```python
from build123d import *

# Parameters (mm, degrees)
BOSS_EXTRUDE1_DEPTH     = 19.05
CUT_EXTRUDE4_DEPTH      = 0.508
CUT_EXTRUDE4_DEPTH_BACK = 6.858
SKETCH4_W               = 31.54
SKETCH4_H               = 60.54
SKETCH4_W_2             = 1.905
SKETCH4_H_2             = 7.62
SKETCH4_3_W             = 1.905
SKETCH4_3_H             = 7.62
CUT_EXTRUDE5_DEPTH      = 34.798
SKETCH5_W               = 31.679207877
SKETCH5_H               = 2.54
SKETCH5_W_2             = 31.841170495
BOSS_EXTRUDE2_DEPTH     = 54.61
SKETCH6_W               = 1.77119272
SKETCH6_H               = 7.149457174
CUT_EXTRUDE6_DEPTH      = 90.782
SKETCH4_5_R             = 1.524
CUT_EXTRUDE7_DEPTH      = 90.782


with BuildPart() as part:
    # Sketch2 → Boss-Extrude1 (new, symmetric)
    with BuildSketch(Plane.XY):
        with BuildLine():
            Line((8.128, -45.72), (8.128, 45.72))
            ThreePointArc((8.128, 45.72), (5.747363917, 51.467363917), (0, 53.848))
            Line((0, 53.848), (0, -53.848))
            ThreePointArc((0, -53.848), (5.747363917, -51.467363917), (8.128, -45.72))
        make_face()
    extrude(amount=BOSS_EXTRUDE1_DEPTH, both=True)

    # Sketch4 → Cut-Extrude4 (cut, two sides: drawn at the far end of the back side and taken through both)
    # profile 1 of 3: a face of its own
    with BuildSketch(Plane.ZY.offset(-CUT_EXTRUDE4_DEPTH_BACK)):
        with Locations((0.025266364, 0.022760685)):
            Rectangle(SKETCH4_W, SKETCH4_H)
        with Locations((-6.375, 9.13)):
            Rectangle(SKETCH4_W_2, SKETCH4_H_2, mode=Mode.SUBTRACT)
        with Locations((6.375, 9.13)):
            Rectangle(SKETCH4_W_2, SKETCH4_H_2, mode=Mode.SUBTRACT)
    # profile 2 of 3: a face of its own
    with BuildSketch(Plane.ZY.offset(-CUT_EXTRUDE4_DEPTH_BACK)):
        with Locations((-6.375, 9.13)):
            Rectangle(SKETCH4_W_2, SKETCH4_H_2)
    # profile 3 of 3: a face of its own
    with BuildSketch(Plane.ZY.offset(-CUT_EXTRUDE4_DEPTH_BACK)):
        with Locations((6.375, 9.13)):
            Rectangle(SKETCH4_W_2, SKETCH4_H_2)
    extrude(amount=CUT_EXTRUDE4_DEPTH + CUT_EXTRUDE4_DEPTH_BACK, mode=Mode.SUBTRACT)

    # Sketch4_3 → Cut-Extrude5 (cut)
    with BuildSketch(Plane.ZY):
        with Locations((-6.375, 9.13)):
            Rectangle(SKETCH4_3_W, SKETCH4_3_H)
        with Locations((6.375, 9.13)):
            Rectangle(SKETCH4_3_W, SKETCH4_3_H)
    extrude(amount=-CUT_EXTRUDE5_DEPTH, mode=Mode.SUBTRACT)

    # Sketch5 → Boss-Extrude2 (add)
    with BuildSketch(Plane.ZY):
        with Locations((0.094870302, -31.517239315)):
            Rectangle(SKETCH5_W, SKETCH5_H)
        with Locations((-0.125318883, 31.562760685)):
            Rectangle(SKETCH5_W_2, SKETCH5_H)
    extrude(amount=BOSS_EXTRUDE2_DEPTH)

    # Sketch6 → Cut-Extrude6 (cut)
    with BuildSketch(Plane(origin=(0, 32.832760685, 0), x_dir=(1, 0, 0), z_dir=(0, 1, 0))):
        with Locations((-50.36366337, 9.522864257)):
            Rectangle(SKETCH6_W, SKETCH6_H)
        with Locations((-50.36366337, -9.522864257)):
            Rectangle(SKETCH6_W, SKETCH6_H)
    extrude(amount=-CUT_EXTRUDE6_DEPTH, mode=Mode.SUBTRACT)

    # Sketch4_5 → Cut-Extrude7 (cut)
    with BuildSketch(Plane.ZY):
        with Locations((16.466357327, -50.756314804)):
            Circle(SKETCH4_5_R)
        with Locations((16.466357327, 50.756314804)):
            Circle(SKETCH4_5_R)
        with Locations((-16.466357327, 50.756314804)):
            Circle(SKETCH4_5_R)
        with Locations((-16.466357327, -50.756314804)):
            Circle(SKETCH4_5_R)
    extrude(amount=-CUT_EXTRUDE7_DEPTH, mode=Mode.SUBTRACT)


solid = part.part
```
Work out the finished part from the listing and answer in its coordinate system (mm). A direction names the side the tool comes from. Round coordinates to 2 decimals unless told otherwise and drop trailing zeros. Write each loop counter-clockwise with the first axis right and the second up, starting at its lowest first coordinate (ties: lowest second). Pieces come first, ordered by that corner, then holes. Notation, with made-up numbers: (63, 13) - (97, 13) arc R33 cw to (97, 41) - close; hole circle Ø11 at (-23, 68). An arc over 180 degrees is marked (long way). Return JSON: item names as keys, results as strings. Group by question number.
Q1. Find the intervals of material crossed by L1, parallel to Y at x = -10, z = 5; L2, parallel to X at y = 31, z = 7; L3, parallel to X at y = -1.5, z = -0.5, in increasing order.
Q2. The part is cut by section D-D on z = 2.5. Write down the section's boundary in (x, y).
Q3. The part is cut by section A-A on z = -8.5. Write down the section's boundary in (x, y).
Q4. The mould has two halves that part along X. Classify faces 1 (the flat face through (-54.61, -31, 0)), 2 (the flat face through (-23, 30.293, 0)), 3 (the flat face through (-51.249, -31, -9)): released by +X, released by -X, zero draft, split by the parting line, or undercut.
Q5. The part is cut by section C-C on y = -26. Write down the section's boundary in (x, z), then the cut area to 3 significant figures.
Q6. For faces 4 (the flat face through (-27, 32.833, 0)), 5 (the flat face through (-49.478, 32, -9)), 6 (the flat face through (-27, 32, -16.046)), 7 (the flat face through (-27, 32, 15.795)), 8 (the flat face through (3, 0, 15.795)), determine the directions among +Z, -Z, +X, -X, +Y, -Y from which every point of the face is accessible in a straight line to the end or side of a thin tool.
Q7. Each of these flat-tipped pins is pushed along its axis until it touches: pin 1 Ø9.5 at (x, z) = (-17.5, 1.5) entering from +Y; pin 2 Ø1.4 at (x, z) = (7.5, -6.5) entering from -Y; pin 3 Ø0.5 at (x, y) = (-50, 32) entering from +Z; pin 4 Ø4 at (x, z) = (0.5, -4.5) entering from +Y. Where does it stop, or does it pass through?
Q8. The part is cut by section B-B on x = -36.5. Write down the section's boundary in (y, z).
Solved:
{
 "1": {"L1": "-32.79 to -30.25, 30.29 to 32.83", "L2": "-54.61 to -51.25, -49.48 to 8.13", "L3": "6.86 to 8.13"},
 "2": {"outline": "(-54.61, -32.79) - (0, -32.79) - (0, -53.85) arc R8.13 ccw to (8.13, -45.72) - (8.13, 45.72) arc R8.13 ccw to (0, 53.85) - (0, 32.83) - (-54.61, 32.83) - (-54.61, 30.29) - (6.86, 30.29) - (6.86, -30.25) - (-54.61, -30.25) - close"},
 "3": {"outline": "(-54.61, -32.79) - (-51.25, -32.79) - (-51.25, -30.25) - (-54.61, -30.25) - close; (-54.61, 30.29) - (-51.25, 30.29) - (-51.25, 32.83) - (-54.61, 32.83) - close; (-49.48, -32.79) - (0, -32.79) - (0, -53.85) arc R8.13 ccw to (8.13, -45.72) - (8.13, 45.72) arc R8.13 ccw to (0, 53.85) - (0, 32.83) - (-49.48, 32.83) - (-49.48, 30.29) - (6.86, 30.29) - (6.86, -30.25) - (-49.48, -30.25) - close"},
 "4": {"face 1": "released by -X", "face 2": "zero draft", "face 3": "undercut"},
 "5": {"outline": "(0, -19.05) - (8.13, -19.05) - (8.13, 19.05) - (0, 19.05) - (0, 15.8) - (6.86, 15.8) - (6.86, -15.74) - (0, -15.74) - close", "area": "93.4 mm²"},
 "6": {"face 4": "+Z, -Z, -X, +Y", "face 5": "+Y, -Y", "face 6": "-Z, -X, +Y, -Y", "face 7": "+Z, -X, +Y", "face 8": "-X"},
 "7": {"pin 1": "y = 32.83", "pin 2": "y = -50.17", "pin 3": "z = 15.8", "pin 4": "y = 53.85"},
 "8": {"outline": "(-32.79, -15.74) - (-30.25, -15.74) - (-30.25, 15.93) - (-32.79, 15.93) - close; (30.29, -16.05) - (32.83, -16.05) - (32.83, 15.8) - (30.29, 15.8) - close"}
}
